from build123d import *

# Parameters (mm, degrees)
SKETCH_1_R      = 14
SKETCH_1_R_2    = 1.5
EXTRUDE_1_DEPTH = 3
EXTRUDE_2_DEPTH = 8


with BuildPart() as part:
    # 草图1 → 凸台-拉伸1 (new body)
    with BuildSketch(Plane.XY):
        Circle(SKETCH_1_R)
        with Locations((0, 10)):
            Circle(SKETCH_1_R_2, mode=Mode.SUBTRACT)
        with Locations((10, 0)):
            Circle(SKETCH_1_R_2, mode=Mode.SUBTRACT)
        with Locations((0, -10)):
            Circle(SKETCH_1_R_2, mode=Mode.SUBTRACT)
        with Locations((-10, 0)):
            Circle(SKETCH_1_R_2, mode=Mode.SUBTRACT)
    extrude(amount=EXTRUDE_1_DEPTH)

    # 草图3 → 凸台-拉伸2 (add)
    with BuildSketch(Plane.XY.offset(3)):
        with BuildLine():
            Line((6, 3.605551275), (6, -3.605551275))
            ThreePointArc((6, -3.605551275), (0, -7), (-6, -3.605551275))
            Line((-6, -3.605551275), (-6, 3.605551275))
            ThreePointArc((-6, 3.605551275), (0, 7), (6, 3.605551275))
        make_face()
    extrude(amount=EXTRUDE_2_DEPTH)


solid = part.part
The model under review builds one solid part; all positions refer to its coordinate system, in mm. A direction names the side the tool comes from. Coordinates: 2 decimals unless noted, no trailing zeros. Write each loop counter-clockwise with the first axis right and the second up, starting at its lowest first coordinate (ties: lowest second). Pieces come first, ordered by that corner, then holes. Notation, with made-up numbers: (59, 31) - (82, 31) arc R24 ccw to (82, 47) - close; hole circle Ø10 at (-5.75, 73). An arc over 180 degrees is marked (long way). Answer as a JSON object with one key per item and string values. Group by question number.
1. Add section B-B (y = -10). Give the boundary of the cut face in (x, z).
2. Mouldability with a two-part tool opening along Y and no side actions: class faces 4 (the face through (-11.5, 0.07, 1.48)), 5 (the face through (0, 7, 7)), 6 (the face through (12.932, -5.362, 1.479)) as pulls with the +Y half, pulls with the -Y half, needs draft (parallel to the pull), parting line crosses it, or undercut.
3. To check wall thickness, follow probe 1 along Y at (x, z) = (0, 1.65); probe 2 along Z at (x, y) = (-8.25, -0.25); probe 3 along X at (y, z) = (-2.25, 7.25). State the ranges of each line that lie inside material, in increasing order.
4. Add section D-D (z = 2.25). Give the boundary of the cut face in (x, y), plus the area to 3 significant figures.
5. Add section A-A (y = 0). Give the boundary of the cut face in (x, z), plus the area to 3 significant figures.
6. Machinability: for faces 1 (the face through (6, 0, 7)), 2 (the face through (0, -7, 7)), 3 (the face through (-6, 0, 7)), which of the approach directions +Z, -Z, +X, -X, +Y, -Y give a long, thin tool a straight path to every point of the face, cutting with its end or side? Answer none if there is none.
7. Clearance check with flat-ended pins moving along their axes: pin 1 Ø1 at (y, z) = (4, 7) entering from +X; pin 2 Ø2 at (x, z) = (-6.5, 9.5) entering from -Y; pin 3 Ø3 at (x, y) = (9.5, 2) entering from +Z. State where each tip first meets the part, or that it passes through.
Findings:
{
 "1": {"outline": "(-9.8, 0) - (-1.5, 0) - (-1.5, 3) - (-9.8, 3) - close; (1.5, 0) - (9.8, 0) - (9.8, 3) - (1.5, 3) - close"},
 "2": {"face 4": "undercut", "face 5": "pulls with the +Y half", "face 6": "parting line crosses it"},
 "3": {"probe 1": "-14 to -11.5, -8.5 to 8.5, 11.5 to 14", "probe 2": "0 to 3", "probe 3": "-6 to 6"},
 "4": {"outline": "circle Ø28 at (0, 0); hole circle Ø3 at (-10, 0); hole circle Ø3 at (0, -10); hole circle Ø3 at (0, 10); hole circle Ø3 at (10, 0)", "area": "587 mm²"},
 "5": {"outline": "(-14, 0) - (-11.5, 0) - (-11.5, 3) - (-14, 3) - close; (-8.5, 0) - (8.5, 0) - (8.5, 3) - (6, 3) - (6, 11) - (-6, 11) - (-6, 3) - (-8.5, 3) - close; (11.5, 0) - (14, 0) - (14, 3) - (11.5, 3) - close", "area": "162 mm²"},
 "6": {"face 1": "+Z, +X, +Y, -Y", "face 2": "+Z, -Y", "face 3": "+Z, -X, +Y, -Y"},
 "7": {"pin 1": "x = 6", "pin 2": "y = -4.33", "pin 3": "z = 3"}
}
